Design review of the part shown in the three views and the two pictorial views. Dimensions are in mm from the part's minimum x, y and z. A direction names the side the tool comes from. Round coordinates to 2 decimals unless told otherwise and drop trailing zeros. Loops run counter-clockwise (first coordinate to the right, second up) from the corner with the lowest first, then second, coordinate; pieces in that order, holes last. Notation, with made-up numbers: (-6.75, 40.25) -> (41.25, 40.25) arc R18 ccw to (41.25, 73.25) -> close; hole circle Ø11 at (65, 76.25). An arc over 180 degrees is marked (long way). Use CSV: the item, a comma, the result in double quotes. Start each with the question number.
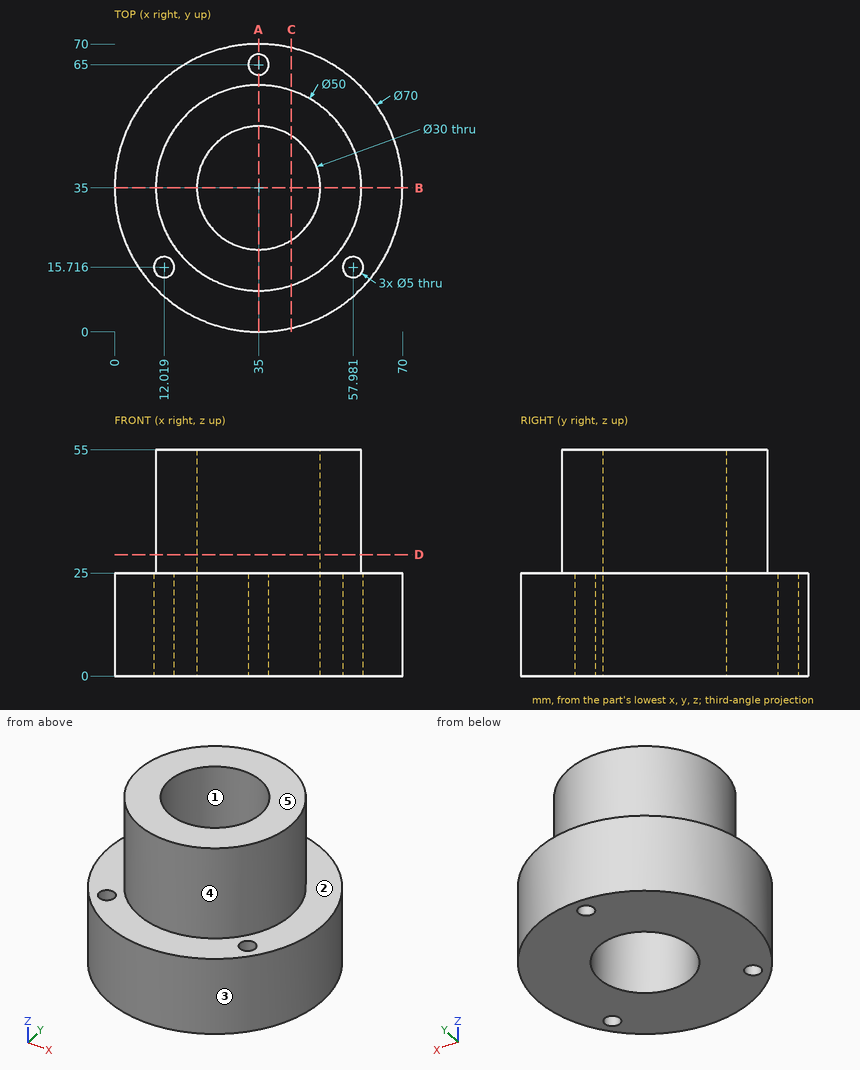
1. The part is to be moulded in two halves that separate along X. For the marked faces 1, 2 and 3, say which applies: pulls with the +X half, pulls with the -X half, needs draft (parallel to the pull), parting line crosses it, or undercut.
2. For line 1 along Y through (x, z) = (35, 23); line 2 along Y through (x, z) = (35, 31); line 3 along Z through (x, y) = (10, 50), list the stretches that pass through material, from the lowest coordinate up. Write a range as from..to.
3. Clearance check with flat-ended pins moving along their axes: P1, Ø1.5, axis at x = 52.5, z = 44.5, coming from the +Y side; P2, Ø6, axis at x = 12.02, y = 15.72, coming from the +Z side; P3, Ø4, axis at x = 55, z = 45.5, coming from the +Y side. State where each tip first meets the part, or that it passes through.
4. Take a section at C-C, the plane x = 43. Give the boundary of the cut face in (y, z) (1 decimal).
5. Take a section at B-B, the plane y = 35. Give the boundary of the cut face in (x, z).
6. Take a section at D-D, the plane z = 29.5. Give the boundary of the cut face in (x, y).
7. Take a section at A-A, the plane x = 35. Give the boundary of the cut face in (y, z), then the cut area to 4 significant figures.
8. For the marked faces 4 and 5, list the 3-axis set-ups (+Z, -Z, +X, -X, +Y, -Y) from which the entire face can be reached by the end or side of a thin tool; tool diameter is ignored.
Results:
1,face 1,"undercut"
1,face 2,"needs draft"
1,face 3,"parting line crosses it"
2,line 1,"0..20, 50..62.5, 67.5..70"
2,line 2,"10..20, 50..60"
2,line 3,"0..25"
3,P1,"y = 53.56"
3,P2,"z = 25"
3,P3,"y = 52.35"
4,outline,"(0.9, 0) -> (22.3, 0) -> (22.3, 55) -> (11.3, 55) -> (11.3, 25) -> (0.9, 25) -> close; (47.7, 0) -> (69.1, 0) -> (69.1, 25) -> (58.7, 25) -> (58.7, 55) -> (47.7, 55) -> close"
5,outline,"(0, 0) -> (20, 0) -> (20, 55) -> (10, 55) -> (10, 25) -> (0, 25) -> close; (50, 0) -> (70, 0) -> (70, 25) -> (60, 25) -> (60, 55) -> (50, 55) -> close"
6,outline,"circle Ø50 at (35, 35); hole circle Ø30 at (35, 35)"
7,outline,"(0, 0) -> (20, 0) -> (20, 55) -> (10, 55) -> (10, 25) -> (0, 25) -> close; (50, 0) -> (62.5, 0) -> (62.5, 25) -> (60, 25) -> (60, 55) -> (50, 55) -> close; (67.5, 0) -> (70, 0) -> (70, 25) -> (67.5, 25) -> close"
7,area,"1,475 mm²"
8,face 4,"+Z"
8,face 5,"+Z, +X, -X, +Y, -Y"
